Could you check a few things on this model? Use its own coordinates, in mm. A direction names the side the tool comes from. Round coordinates to 2 decimals unless told otherwise and drop trailing zeros. Order: outer loops, then holes, each group sorted by start corner. A loop starts at its lowest first (then second) coordinate and runs counter-clockwise, first axis right, second up.
Autodesk Inventor part; units mm, degrees
ref_plane "YZ Plane" through (0, 0, 0) normal (1, 0, 0) x (0, 1, 0)
ref_plane "XZ Plane" through (0, 0, 0) normal (0, 1, 0) x (-1, 0, 0)
ref_plane "XY Plane" through (0, 0, 0) normal (0, 0, 1) x (1, 0, 0)
sketch "Sketch1" plane through (0, 0, 0) normal (0, 0, 1) x (1, 0, 0)
  line L0 (0, 4) -> (0, 26)
  line L1 (0, 26) -> (20, 26)
  line L2 (20, 26) -> (20, 30)
  line L3 (20, 30) -> (30, 30)
  line L4 (30, 30) -> (30, 26)
  line L5 (30, 26) -> (45, 26)
  line L6 (45, 26) -> (45, 30)
  line L7 (45, 30) -> (55, 30)
  line L8 (55, 30) -> (55, 26)
  line L9 (55, 26) -> (70, 26)
  line L10 (70, 26) -> (70, 30)
  line L11 (70, 30) -> (80, 30)
  line L12 (80, 30) -> (80, 26)
  line L13 (80, 26) -> (100, 26)
  line L14 (100, 26) -> (100, 4)
  line L15 (100, 4) -> (80, 4)
  line L16 (80, 4) -> (80, 0)
  line L17 (80, 0) -> (70, 0)
  line L18 (70, 0) -> (70, 4)
  line L19 (55, 4) -> (70, 4)
  line L20 (55, 4) -> (55, 0)
  line L21 (45, 0) -> (45, 4)
  line L22 (30, 4) -> (30, 0)
  line L23 (45, 4) -> (30, 4)
  line L24 (45, 0) -> (55, 0)
  line L25 (30, 0) -> (20, 0)
  line L26 (20, 4) -> (20, 0)
  line L27 (20, 4) -> (0, 4)
  point P0 (0, 0)
  dimension "d0" = 22
  dimension "d1" = 20
  dimension "d2" = 4
  dimension "d3" = 10
  dimension "d4" = 15
  dimension "d5" = 10
  dimension "d6" = 15
  dimension "d7" = 10
  dimension "d8" = 20
  dimension "d9" = 22
  dimension "d10" = 20
extrude "Extrusion1" add sketch "Sketch1" along normal blind 4
sketch "Sketch2" plane through (0, 0, 4) normal (0, 0, 1) x (1, 0, 0)
  line L0 (50, 20.5) -> (40.25, 20.5)
  line L1 (40.25, 20.5) -> (59.75, 20.5)
  line L2 (50, 15) -> (58.5, 15)
  line L3 (58.5, 15) -> (41.5, 15)
  line L4 (41.5, 15) -> (40.25, 20.5)
  line L5 (58.5, 15) -> (59.75, 20.5)
  point P0 (0, 0)
  dimension "d19" = 5.5
  dimension "d20" = 9.75
extrude "Extrusion2" cut sketch "Sketch2" against normal blind 4
properties part number "front(vga)"
Q1. We'd pull the mould along X, two halves only. Please class faces 1 (the flat face through (49, 12, 4)), 2 (the flat face through (0, 15, 2)), 3 (the flat face through (45, 28, 2)): released by +X, released by -X, zero draft, split by the parting line, or undercut.
Q2. I need wall thicknesses on L1, parallel to X at y = 28, z = 2.15; L2, parallel to Y at x = 88, z = 3.85; L3, parallel to X at y = 17.75, z = 2.6 (3 decimals). Which ranges of each line are inside material? Lowest first, please.
Q3. For faces 4 (the flat face through (40.884, 17.711, 2.028)), 5 (the flat face through (20, 28, 2)), 6 (the flat face through (80, 28, 2)), which set-ups out of +Z, -Z, +X, -X, +Y, -Y let a thin tool reach every point of the face, with its end or its side?
Q4. For P1, Ø2, axis at y = 27.5, z = 2.5, coming from the -X side; P2, Ø1.2, axis at y = 1.5, z = 1, coming from the +X side; P3, Ø4, axis at x = 12, y = 8.5, coming from the -Z side; P4, Ø2, axis at x = 38, z = 3, coming from the +Y side, each with a flat end and sliding along its axis, tell me the tip position at first contact or that it passes through.
Q5. Imagine slicing it at A-A, the plane x = 49.5. Please give me the cut outline in (y, z).
Q6. Imagine slicing it at C-C, the plane x = 69. Please give me the cut outline in (y, z), then the cut area to 3 significant figures.
Filled in:
1. face 1: zero draft
1. face 2: released by -X
1. face 3: undercut
2. L1: x = 20 to 30, 45 to 55, 70 to 80
2. L2: y = 4 to 26
2. L3: x = 0 to 40.875, 59.125 to 100
3. face 4: +Z, -Z
3. face 5: +Z, -Z, -X, +Y
3. face 6: +Z, -Z, +X, +Y
4. P1: stops at x = 20
4. P2: stops at x = 80
4. P3: stops at z = 0
4. P4: stops at y = 26
5. outline: (0, 0) - (15, 0) - (15, 4) - (0, 4) - close; (20.5, 0) - (30, 0) - (30, 4) - (20.5, 4) - close
6. outline: (4, 0) - (26, 0) - (26, 4) - (4, 4) - close
6. area: 88.0 mm2
